from build123d import *

# Parameters (mm, degrees)
SKETCH1_R           = 2.54
SKETCH1_R_2         = 2.0193
SKETCH1_R_3         = 9.525
BOSS_EXTRUDE1_DEPTH = 4.7625


with BuildPart() as part:
    # Sketch1 → Boss-Extrude1 (new body)
    with BuildSketch(Plane(origin=(0, 0, 0), x_dir=(0, 0, -1), z_dir=(1, 0, 0))):
        with BuildLine():
            Line((226.734866781, 43.274288567), (226.734866781, 106.774288567))
            ThreePointArc((226.734866781, 106.774288567), (230.45461066, 115.754544688), (239.434866781, 119.474288567))
            Line((239.434866781, 119.474288567), (391.834866781, 119.474288567))
            ThreePointArc((391.834866781, 119.474288567), (400.815122902, 115.754544688), (404.534866781, 106.774288567))
            Line((404.534866781, 106.774288567), (404.534866781, 43.274288567))
            ThreePointArc((404.534866781, 43.274288567), (400.815122902, 34.294032445), (391.834866781, 30.574288567))
            Line((391.834866781, 30.574288567), (239.434866781, 30.574288567))
            ThreePointArc((239.434866781, 30.574288567), (230.45461066, 34.294032445), (226.734866781, 43.274288567))
        make_face()
        with Locations(Location((302.934866781, 111.854288567, 0), (0, 0, 180))):
            Circle(SKETCH1_R, mode=Mode.SUBTRACT)
        with Locations(Location((328.334866781, 111.854288567, 0), (0, 0, 180))):
            Circle(SKETCH1_R, mode=Mode.SUBTRACT)
        with Locations(Location((315.634866781, 100.424288567, 0), (0, 0, 180))):
            Circle(SKETCH1_R_2, mode=Mode.SUBTRACT)
        with Locations(Location((302.934866781, 38.194288567, 0), (0, 0, 180))):
            Circle(SKETCH1_R, mode=Mode.SUBTRACT)
        with Locations(Location((328.334866781, 38.194288567, 0), (0, 0, 180))):
            Circle(SKETCH1_R, mode=Mode.SUBTRACT)
        with Locations(Location((239.434866781, 43.274288567, 0), (0, 0, 180))):
            Circle(SKETCH1_R, mode=Mode.SUBTRACT)
        with Locations(Location((391.834866781, 43.274288567, 0), (0, 0, 180))):
            Circle(SKETCH1_R, mode=Mode.SUBTRACT)
        with Locations(Location((315.634866781, 75.024288567, 0), (0, 0, 180))):
            Circle(SKETCH1_R_3, mode=Mode.SUBTRACT)
        with Locations(Location((315.634866781, 49.624288567, 0), (0, 0, 180))):
            Circle(SKETCH1_R_2, mode=Mode.SUBTRACT)
        with Locations(Location((239.434866781, 106.774288567, 0), (0, 0, 180))):
            Circle(SKETCH1_R, mode=Mode.SUBTRACT)
        with Locations(Location((391.834866781, 106.774288567, 0), (0, 0, 180))):
            Circle(SKETCH1_R, mode=Mode.SUBTRACT)
        with Locations(Location((269.914866781, 75.024288567, 0), (0, 0, 180))):
            Circle(SKETCH1_R_3, mode=Mode.SUBTRACT)
        with Locations(Location((361.354866781, 75.024288567, 0), (0, 0, 180))):
            Circle(SKETCH1_R_3, mode=Mode.SUBTRACT)
    extrude(amount=BOSS_EXTRUDE1_DEPTH)


with BuildPart() as part_1:
    # Body-Move/Copy1: moved
    add(part.part.moved(Location((0, 0, 631.269733563))))


solid = part_1.part
Geometry: final body of the model. Coordinates: model frame, mm. Give positions to 0.01 mm unless a question says otherwise; leave off trailing zeros. Loops run counter-clockwise (first coordinate to the right, second up) from the corner with the lowest first, then second, coordinate; pieces in that order, holes last. Notation, with made-up numbers: M -9.5,20 L 24.5,20 A28 ccw 24.5,51 Z; hole C 47.5,16 d10. An arc over 180 degrees is marked long. Put each result on its own line as item: value.
1) Cut plane A-A, the plane z = 320.5. Return the cut outline in (x, y).
Computed values:
outline: M 0,30.57 L 4.76,30.57 L 4.76,66.84 L 0,66.84 Z; M 0,83.21 L 4.76,83.21 L 4.76,119.47 L 0,119.47 Z
2) First-contact query: P1, Ø1.5, axis at y = 86.5, z = 346, coming from the -X side; P2, Ø4, axis at y = 106.77, z = 239.43, coming from the +X side. Flat tips, straight axial feed; report the tip coordinate or a pass-through.
Computed values:
P1: stops at x = 0
P2: passes through
3) Material intervals for L1, parallel to Z at x = 3.65, y = 75.5; L2, parallel to Z at x = 1.8, y = 71.5; L3, parallel to Z at x = 2.3, y = 111, sorted ascending. Write a range as from..to.
Computed values:
L1: z = 226.73..260.4, 279.43..306.12, 325.15..351.84, 370.87..404.53
L2: z = 226.73..261.07, 278.76..306.79, 324.48..352.51, 370.2..404.53
L3: z = 227.46..300.54, 305.33..325.94, 330.73..403.81
4) Cut plane B-B, the plane x = 2.6. Give the number of separate pieces and of enclosed holes in the cut face, plus the area to 3 significant figures.
Computed values:
separate pieces: 1
enclosed holes: 13
area: 14,600 mm^2
5) Cut plane C-C, the plane z = 273.5. Return the cut outline in (x, y), plus the area to 3 significant figures.
Computed values:
outline: M 0,30.57 L 4.76,30.57 L 4.76,66.2 L 0,66.2 Z; M 0,83.85 L 4.76,83.85 L 4.76,119.47 L 0,119.47 Z
area: 339 mm^2
6) Mould query, pull axis Y, two halves, no side actions, for faces 1 (the cylindrical face through (2.3, 44.2, 241.8)), 2 (the cylindrical face through (2.35, 34.39, 230.36)), 3 (the flat face through (2, 119.474, 317)). Classes: released by +Y, released by -Y, zero draft, split by the parting line, or undercut.
Computed values:
face 1: undercut
face 2: released by -Y
face 3: released by +Y
